Source: CAD feature listing. Evaluate the final solid. Frame: model axes, mm. A direction names the side the tool comes from. Give positions to 0.01 mm unless a question says otherwise; leave off trailing zeros. Order: outer loops, then holes, each group sorted by start corner. A loop starts at its lowest first (then second) coordinate and runs counter-clockwise, first axis right, second up. Notation, with made-up numbers: (63, 14.25) -> (78, 14.25) arc R28 cw to (78, 49.25) -> close; hole circle Ø5 at (-26.5, 16). An arc over 180 degrees is marked (long way). Answer in a Markdown table with one row per item.
```python
from build123d import *

# Parameters (mm, degrees)
F0_W      = 25
F0_H      = 25
F0_R      = 1.5
F1_DEPTH  = 3
F2_DEPTH  = 3
F3_W      = 25
F3_H      = 3
F4_DEPTH  = 22
F5_W      = 3
F5_H      = 22
F6_DEPTH  = 22
F8_DEPTH  = 25
F9_R      = 5
F10_DEPTH = 25


with BuildPart() as f1:
    # F0 (on Top) → F1 (new body)
    with BuildSketch(Plane.XY):
        with Locations((2.5, -4.5)):
            Rectangle(F0_W, F0_H)
        with Locations((-7, 0)):
            Circle(F0_R, mode=Mode.SUBTRACT)
        with BuildLine():
            ThreePointArc((4.5, 0), (3, -1.5), (1.5, 0))
            ThreePointArc((1.5, 0), (3, 1.5), (4.5, 0))
        make_face(mode=Mode.SUBTRACT)
    extrude(amount=F1_DEPTH)

    # F0 (on Top) → F2 (join)
    with BuildSketch(Plane.XY):
        with Locations((2.5, -4.5)):
            Rectangle(F0_W, F0_H)
        with Locations((-7, 0)):
            Circle(F0_R, mode=Mode.SUBTRACT)
        with BuildLine():
            ThreePointArc((4.5, 0), (3, -1.5), (1.5, 0))
            ThreePointArc((1.5, 0), (3, 1.5), (4.5, 0))
        make_face(mode=Mode.SUBTRACT)
    extrude(amount=F2_DEPTH)

    # F3 (on face) → F4 (join)
    with BuildSketch(Plane.XY.offset(3)):
        with Locations((2.5, -15.5)):
            Rectangle(F3_W, F3_H)
    extrude(amount=F4_DEPTH)

    # F5 (on face) → F6 (join)
    with BuildSketch(Plane(origin=(0, -14, 0), x_dir=(-1, 0, 0), z_dir=(0, 1, 0))):
        with Locations((-13.5, 14)):
            Rectangle(F5_W, F5_H)
    extrude(amount=F6_DEPTH)

    # F7 (on face) → F8 (cut)
    with BuildSketch(Plane(origin=(12, 0, 0), x_dir=(0, -1, 0), z_dir=(-1, 0, 0))):
        with BuildLine():
            ThreePointArc((1.5, 12), (1.06066, 13.06066), (0, 13.5))
            ThreePointArc((0, 13.5), (-1.06066, 10.93934), (1.5, 12))
        make_face()
        with BuildLine():
            Line((0, 22), (0, 23.5))
            ThreePointArc((0, 23.5), (-1.5, 22), (0, 20.5))
            Line((0, 20.5), (0, 22))
        make_face()
        with BuildLine():
            ThreePointArc((0, 20.5), (1.06066, 20.93934), (1.5, 22))
            ThreePointArc((1.5, 22), (1.06066, 23.06066), (0, 23.5))
            Line((0, 23.5), (0, 22))
            Line((0, 22), (0, 20.5))
        make_face()
    extrude(amount=-F8_DEPTH, mode=Mode.SUBTRACT)

    # F9 (on face) → F10 (cut)
    with BuildSketch(Plane.XZ.offset(17)):
        with Locations((0, 15)):
            Circle(F9_R)
    extrude(amount=-F10_DEPTH, mode=Mode.SUBTRACT)


solid = f1.part
```
(1) Section query A-A (z = 18). Return the cut outline in (x, y), plus the area to 3 significant figures.
A:
| item | result |
|---|---|
| outline | (-10, -17) -> (-4, -17) -> (-4, -14) -> (-10, -14) -> close; (4, -17) -> (15, -17) -> (15, 8) -> (12, 8) -> (12, -14) -> (4, -14) -> close |
| area | 117 mm^2 |
(2) Section query C-C (y = -0.5). Return the cut outline in (x, z).
A:
| item | result |
|---|---|
| outline | (-10, 0) -> (-8.41, 0) -> (-8.41, 3) -> (-10, 3) -> close; (-5.59, 0) -> (1.59, 0) -> (1.59, 3) -> (-5.59, 3) -> close; (4.41, 0) -> (15, 0) -> (15, 10.59) -> (12, 10.59) -> (12, 3) -> (4.41, 3) -> close; (12, 13.41) -> (15, 13.41) -> (15, 20.59) -> (12, 20.59) -> close; (12, 23.41) -> (15, 23.41) -> (15, 25) -> (12, 25) -> close |
(3) Pull-direction query (Y, two-part tool) for faces 1 (the cylindrical face through (1.57, 0.45, 1.48)), 2 (the cylindrical face through (-1.08, -15.52, 10.12)), 3 (the flat face through (1, -14, 9)); classes: +Y half, -Y half, draft (parallel to the pull), parting line (faces both ways), or undercut.
A:
| item | result |
|---|---|
| face 1 | undercut |
| face 2 | draft |
| face 3 | +Y half |
(4) Ray query, probe 1 along Z at (x, y) = (13.7, 0); probe 2 along Y at (x, z) = (-7, 1.7); probe 3 along Z at (x, y) = (-1.25, -13.75). Return the intervals inside material, ascending.
A:
| item | result |
|---|---|
| probe 1 | z = 0 to 10.5, 13.5 to 20.5, 23.5 to 25 |
| probe 2 | y = -17 to -1.5, 1.5 to 8 |
| probe 3 | z = 0 to 3 |
(5) Section query D-D (x = -7). Return the cut outline in (y, z).
A:
| item | result |
|---|---|
| outline | (-17, 0) -> (-1.5, 0) -> (-1.5, 3) -> (-14, 3) -> (-14, 25) -> (-17, 25) -> close; (1.5, 0) -> (8, 0) -> (8, 3) -> (1.5, 3) -> close |
(6) First-contact query: pin 1 Ø4 at (y, z) = (-3.5, 11) entering from -X; pin 2 Ø2.5 at (x, y) = (3, 0) entering from +Z; pin 3 Ø10 at (x, z) = (-1, 10) entering from +Y; pin 4 Ø4 at (x, y) = (-7, 0) entering from +Z. Flat tips, straight axial feed; report the tip coordinate or a pass-through.
A:
| item | result |
|---|---|
| pin 1 | stops at x = 12 |
| pin 2 | passes through |
| pin 3 | stops at y = -14 |
| pin 4 | stops at z = 3 |
(7) Section query B-B (x = 3). Return the cut outline in (y, z), plus the area to 3 significant figures.
A:
| item | result |
|---|---|
| outline | (-17, 0) -> (-1.5, 0) -> (-1.5, 3) -> (-14, 3) -> (-14, 11) -> (-17, 11) -> close; (-17, 19) -> (-14, 19) -> (-14, 25) -> (-17, 25) -> close; (1.5, 0) -> (8, 0) -> (8, 3) -> (1.5, 3) -> close |
| area | 108 mm^2 |
(8) Access query for faces 4 (the cylindrical face through (-8.5, 0.07, 1.48)), 5 (the flat face through (12, -3, 14)). Directions: +Z, -Z, +X, -X, +Y, -Y. A direction counts if a zero-diameter tool reaches every point of the face in a straight line with its end or side. Return the directions, or none.
A:
| item | result |
|---|---|
| face 4 | +Z, -Z |
| face 5 | +Z, -X, +Y |
